Read the model definition and answer for the solid it produces. Units are mm, in the model's axes. Face numbers are marked on the shaded views. A direction names the side the tool comes from. Give positions to 0.01 mm unless a question says otherwise; leave off trailing zeros. Write each loop counter-clockwise with the first axis right and the second up, starting at its lowest first coordinate (ties: lowest second). Pieces come first, ordered by that corner, then holes. Notation, with made-up numbers: (33.25, 5.25) - (90.25, 5.25) arc R19 cw to (90.25, 34.25) - close; hole circle Ø9 at (0.5, 87.5). An arc over 180 degrees is marked (long way). Answer as CSV lines item,"result".
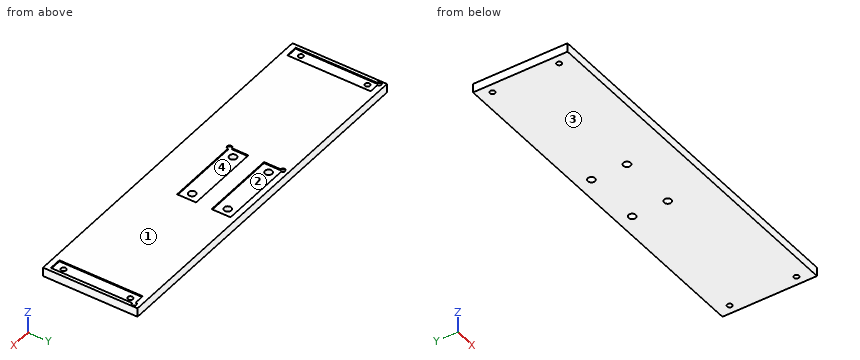
```python
from build123d import *

# Parameters (mm, degrees)
ESQUISSE1_W             = 324
ESQUISSE1_H             = 85
BOSS_EXTRU_1_DEPTH      = 8
ENL_V_MAT_EXTRU_1_DEPTH = 1
ESQUISSE3_R             = 2.25
ENL_V_MAT_EXTRU_2_DEPTH = 168.628309065
ENL_V_MAT_EXTRU_3_DEPTH = 1
ESQUISSE5_R             = 3.25
ENL_V_MAT_EXTRU_4_DEPTH = 168.628309065


with BuildPart() as part:
    # Esquisse1 → Boss.-Extru.1 (new body)
    with BuildSketch(Plane.XY):
        Rectangle(ESQUISSE1_W, ESQUISSE1_H)
    extrude(amount=BOSS_EXTRU_1_DEPTH)

    # Esquisse2 → Enlèv. mat.-Extru.1 (cut)
    with BuildSketch(Plane.XY.offset(8)):
        with BuildLine():
            Line((148, 37.5), (156.9, 37.5))
            ThreePointArc((156.9, 37.5), (160.48492424, 38.98492424), (159, 35.4))
            Line((159, 35.4), (159, -37.5))
            Line((159, -37.5), (148, -37.5))
            Line((148, -37.5), (148, 37.5))
        make_face()
    enl_v_mat_extru_1 = extrude(amount=-ENL_V_MAT_EXTRU_1_DEPTH, mode=Mode.SUBTRACT)

    # Symétrie1: Enlèv. mat.-Extru.1 across plane
    add(enl_v_mat_extru_1.mirror(Plane(origin=(0, 0, 0), x_dir=(0, 0, 1), z_dir=(1, 0, 0))), mode=Mode.SUBTRACT)

    # Esquisse3 → Enlèv. mat.-Extru.2 (cut, through all)
    with BuildSketch(Plane.XY.offset(7)):
        with Locations((154, 30.5)):
            Circle(ESQUISSE3_R)
        with Locations(Location((154, -29.5, 0), (0, 0, 180))):
            Circle(ESQUISSE3_R)
    enl_v_mat_extru_2 = extrude(amount=-ENL_V_MAT_EXTRU_2_DEPTH, mode=Mode.SUBTRACT)

    # Symétrie2: Enlèv. mat.-Extru.2 across plane
    add(enl_v_mat_extru_2.mirror(Plane(origin=(0, 0, 0), x_dir=(0, 0, 1), z_dir=(1, 0, 0))), mode=Mode.SUBTRACT)

    # Esquisse4 → Enlèv. mat.-Extru.3 (cut)
    with BuildSketch(Plane.XY.offset(8)):
        with BuildLine():
            Line((-31.9, 37.5), (34, 37.5))
            Line((34, 37.5), (34, 20.5))
            Line((34, 20.5), (-34, 20.5))
            Line((-34, 20.5), (-34, 35.4))
            ThreePointArc((-34, 35.4), (-35.48492424, 38.98492424), (-31.9, 37.5))
        make_face()
        with BuildLine():
            Line((34, -10.5), (34, 6.5))
            Line((34, 6.5), (-34, 6.5))
            Line((-34, 6.5), (-34, -8.4))
            ThreePointArc((-34, -8.4), (-35.48492424, -11.98492424), (-31.9, -10.5))
            Line((-31.9, -10.5), (34, -10.5))
        make_face()
    extrude(amount=-ENL_V_MAT_EXTRU_3_DEPTH, mode=Mode.SUBTRACT)

    # Esquisse5 → Enlèv. mat.-Extru.4 (cut, through all)
    with BuildSketch(Plane.XY.offset(7)):
        with Locations((-27, 29.5)):
            Circle(ESQUISSE5_R)
        with Locations(Location((26, 29.5, 0), (0, 0, 180))):
            Circle(ESQUISSE5_R)
        with Locations((26, -2.5)):
            Circle(ESQUISSE5_R)
        with Locations(Location((-27, -2.5, 0), (0, 0, 180))):
            Circle(ESQUISSE5_R)
    extrude(amount=-ENL_V_MAT_EXTRU_4_DEPTH, mode=Mode.SUBTRACT)


solid = part.part
```
(1) A cutting plane is placed at B-B (y = -2.5). Write down the section's boundary in (x, z).
Worked out:
outline,"(-162, 0) - (-30.25, 0) - (-30.25, 7) - (-34, 7) - (-34, 8) - (-148, 8) - (-148, 7) - (-159, 7) - (-159, 8) - (-162, 8) - close; (-23.75, 0) - (22.75, 0) - (22.75, 7) - (-23.75, 7) - close; (29.25, 0) - (162, 0) - (162, 8) - (159, 8) - (159, 7) - (148, 7) - (148, 8) - (34, 8) - (34, 7) - (29.25, 7) - close"
(2) The mould has two halves that part along Y. Classify the marked faces 3 and 4: +Y half, -Y half, draft (parallel to the pull), parting line (faces both ways), or undercut.
Worked out:
face 3,"draft"
face 4,"undercut"
(3) A cutting plane is placed at A-A (x = 26). Write down the section's boundary in (y, z), and give its area (3 significant figures).
Worked out:
outline,"(-42.5, 0) - (-5.75, 0) - (-5.75, 7) - (-10.5, 7) - (-10.5, 8) - (-42.5, 8) - close; (0.75, 0) - (26.25, 0) - (26.25, 7) - (20.5, 7) - (20.5, 8) - (6.5, 8) - (6.5, 7) - (0.75, 7) - close; (32.75, 0) - (42.5, 0) - (42.5, 8) - (37.5, 8) - (37.5, 7) - (32.75, 7) - close"
area,"555 mm^2"
(4) Each of these flat-tipped pins is pushed along its axis until it touches: P1, Ø2.5, axis at x = 159, y = 37.5, coming from the +Z side; P2, Ø4, axis at x = -154, y = 30.5, coming from the +Z side. Where does it stop, or does it pass through?
Worked out:
P1,"stops at z = 7"
P2,"passes through"
(5) For the marked faces 1 and 2, determine the directions among +Z, -Z, +X, -X, +Y, -Y from which every point of the face is accessible in a straight line to the end or side of a thin tool.
Worked out:
face 1,"+Z, +X, -X, +Y, -Y"
face 2,"+Z"
(6) Find the intervals of material crossed by L1, parallel to Y at x = -27, z = 2.75; L2, parallel to X at y = -30, z = 4.25; L3, parallel to X at y = -13, z = 7.75, in increasing order.
Worked out:
L1,"y = -42.5 to -5.75, 0.75 to 26.25, 32.75 to 42.5"
L2,"x = -162 to -156.19, -151.81 to 151.81, 156.19 to 162"
L3,"x = -162 to -159, -148 to 148, 159 to 162"
